from build123d import *

# Parameters (mm, degrees)
F0_W     = 50
F0_H     = 100
F1_DEPTH = 13
F2_W     = 50
F2_H     = 20
F3_DEPTH = 40.2
F4_R     = 10
F5_DEPTH = 66.4


# Not quite as in the source:
# - a feature names something its author has since deleted; it is built from what else it names


with BuildPart() as f1:
    # F0 (on Front) → F1 (new body)
    with BuildSketch(Plane.XZ):
        Rectangle(F0_W, F0_H)
    extrude(amount=F1_DEPTH)

    # F2 (on face) → F3 (join)
    with BuildSketch(Plane.XZ.offset(13)):
        with Locations((0, -40)):
            Rectangle(F2_W, F2_H)
    extrude(amount=F3_DEPTH)

    # F4 (on face) → F5 (cut)
    with BuildSketch(Plane(origin=(0, 0, 0), x_dir=(-1, 0, 0), z_dir=(0, 1, 0))):
        Circle(F4_R)
    extrude(amount=-F5_DEPTH, mode=Mode.SUBTRACT)


solid = f1.part
Source: CAD feature listing. Evaluate the final solid. Frame: model axes, mm. A direction names the side the tool comes from. Coordinates: 2 decimals unless noted, no trailing zeros. Write each loop counter-clockwise with the first axis right and the second up, starting at its lowest first coordinate (ties: lowest second). Pieces come first, ordered by that corner, then holes. Notation, with made-up numbers: M -30.5,-24.5 L -26.5,-24.5 A37 cw -26.5,11.5 Z; hole C 35,-16 d6. An arc over 180 degrees is marked long. Use a Markdown table: item, result.
1) First-contact query: pin 1 Ø12 at (x, z) = (0, 0) entering from -Y; pin 2 Ø3 at (x, z) = (-8.5, 29.5) entering from -Y. Flat tips, straight axial feed; report the tip coordinate or a pass-through.
Conclusion:
| item | result |
|---|---|
| pin 1 | passes through |
| pin 2 | stops at y = -13 |
2) Section B-B, the plane x = 0. Output: boundary loops of the cut face in (y, z), then the cut area to 3 significant figures.
Conclusion:
| item | result |
|---|---|
| outline | M -53.2,-50 L 0,-50 L 0,-10 L -13,-10 L -13,-30 L -53.2,-30 Z; M -13,10 L 0,10 L 0,50 L -13,50 Z |
| area | 1,840 mm^2 |
3) Section D-D, the plane x = 18.5. Output: boundary loops of the cut face in (y, z), then the cut area to 3 significant figures.
Conclusion:
| item | result |
|---|---|
| outline | M -53.2,-50 L 0,-50 L 0,50 L -13,50 L -13,-30 L -53.2,-30 Z |
| area | 2,100 mm^2 |
4) Section A-A, the plane z = -8. Output: boundary loops of the cut face in (x, y), then the cut area to 3 significant figures.
Conclusion:
| item | result |
|---|---|
| outline | M -25,-13 L -6,-13 L -6,0 L -25,0 Z; M 6,-13 L 25,-13 L 25,0 L 6,0 Z |
| area | 494 mm^2 |
5) Mould query, pull axis X, two halves, no side actions, for faces 1 (the cylindrical face through (2.17, -6.41, -9.76)), 2 (the flat face through (-25, -8, -23)), 3 (the flat face through (0, 0, 12)). Classes: pulls with the +X half, pulls with the -X half, needs draft (parallel to the pull), parting line crosses it, or undercut.
Conclusion:
| item | result |
|---|---|
| face 1 | undercut |
| face 2 | pulls with the -X half |
| face 3 | needs draft |
6) Ray query, L1, parallel to Z at x = 0, y = -5; L2, parallel to Y at x = 8.5, z = 33.5; L3, parallel to Z at x = 3, y = -28. Return the intervals inside material, ascending.
Conclusion:
| item | result |
|---|---|
| L1 | z = -50 to -10, 10 to 50 |
| L2 | y = -13 to 0 |
| L3 | z = -50 to -30 |
7) Section C-C, the plane y = -9. Output: boundary loops of the cut face in (x, z).
Conclusion:
| item | result |
|---|---|
| outline | M -25,-50 L 25,-50 L 25,50 L -25,50 Z; hole C 0,0 d20 |
8) Reachability of faces 4 (the flat face through (25, -8, -23)), 5 (the flat face through (0, -13, 11)) from +Z, -Z, +X, -X, +Y, -Y: full face, straight path, thin tool, end or side. Return the list, or none.
Conclusion:
| item | result |
|---|---|
| face 4 | +Z, -Z, +X, +Y, -Y |
| face 5 | +Z, +X, -X, -Y |
